from build123d import *

# Parameters (mm, degrees)
F0_R     = 0.635
F0_R_2   = 1.015
F1_DEPTH = 1.85
F2_W     = 2.096224
F2_H     = 1.321533
F3_DEPTH = 0.95


with BuildPart() as f1:
    # F0 (on Top) → F1 (new body)
    with BuildSketch(Plane.XY):
        with BuildLine():
            ThreePointArc((-2.54, -13.97), (-1.796051, -15.766051), (0, -16.51))
            Line((0, -16.51), (12.7, -16.51))
            ThreePointArc((12.7, -16.51), (14.496051, -15.766051), (15.24, -13.97))
            Line((15.24, -13.97), (15.24, 0))
            ThreePointArc((15.24, 0), (14.496051, 1.796051), (12.7, 2.54))
            Line((12.7, 2.54), (0, 2.54))
            ThreePointArc((0, 2.54), (-1.796051, 1.796051), (-2.54, 0))
            Line((-2.54, 0), (-2.54, -13.97))
        make_face()
        with Locations((-1.27, -13.97)):
            Circle(F0_R, mode=Mode.SUBTRACT)
        with Locations((1.27, -13.97)):
            Circle(F0_R, mode=Mode.SUBTRACT)
        with Locations((3.81, -13.97)):
            Circle(F0_R, mode=Mode.SUBTRACT)
        with Locations((6.35, -13.97)):
            Circle(F0_R, mode=Mode.SUBTRACT)
        with Locations((8.89, -13.97)):
            Circle(F0_R, mode=Mode.SUBTRACT)
        with Locations((11.43, -13.97)):
            Circle(F0_R, mode=Mode.SUBTRACT)
        with Locations((13.97, -13.97)):
            Circle(F0_R, mode=Mode.SUBTRACT)
        Circle(F0_R_2, mode=Mode.SUBTRACT)
        with Locations((12.7, 0)):
            Circle(F0_R_2, mode=Mode.SUBTRACT)
    extrude(amount=F1_DEPTH)

    # F2 (on face) → F3 (join)
    with BuildSketch(Plane.XY.offset(1.85)):
        with Locations((5.915654, -5.278095)):
            Rectangle(F2_W, F2_H)
    extrude(amount=F3_DEPTH)


solid = f1.part
Verification items for the finished model (mm, model axes). A direction names the side the tool comes from. Give positions to 0.01 mm unless a question says otherwise; leave off trailing zeros. Write each loop counter-clockwise with the first axis right and the second up, starting at its lowest first coordinate (ties: lowest second). Pieces come first, ordered by that corner, then holes. Notation, with made-up numbers: M -4,-24.5 L 11,-24.5 A25 ccw 11,1.5 Z; hole C 77.25,-13 d11. An arc over 180 degrees is marked long. Put each result on its own line as item: value. Start each with the question number.
1. Section check C-C (y = -0.25). Record the cut outline in (x, z), and give its area (3 significant figures).
2. Section check B-B (z = 0.8). Give the number of separate pieces and of enclosed holes in the cut face, and give its area (3 significant figures).
3. Set-up check for faces 5 (the face through (4.868, -5, 2)), 6 (the face through (5.9, -4.617, 2.3)), 7 (the face through (5.9, -5.939, 2.3)): record each of +Z, -Z, +X, -X, +Y, -Y from which the full face is reachable in a straight line by a thin tool's end or side.
4. Go/stop test with flat-tipped pins: pin 1 Ø2.5 at (x, y) = (12.7, 0) entering from +Z; pin 2 Ø1.2 at (x, y) = (0, 0) entering from -Z; pin 3 Ø1 at (x, z) = (5.5, 2.5) entering from -Y; pin 4 Ø0.5 at (y, z) = (-5.5, 2.5) entering from -X. Record where each tip stops, or that it passes through.
5. Scan lines: line 1 along Y through (x, z) = (3.81, 1.4) (3 decimals); line 2 along Z through (x, y) = (2.75, -12.75); line 3 along Y through (x, z) = (14.5, 0.4). Record each from-to range of solid material in increasing order. Write a range as [from, to].
6. Section check D-D (x = 9.25). Record the cut outline in (y, z).
7. Section check A-A (x = 1.27). Record the cut outline in (y, z) (3 decimals).
8. Draft check along Y on faces 1 (the face through (-2.54, -7, 1)), 2 (the face through (-1.776, 1.816, 0.912)), 3 (the face through (-1.35, -13.34, 0.91)), 4 (the face through (6.691, -13.435, 0.912)). Enter one of: +Y half, -Y half, draft (parallel to the pull), parting line (faces both ways), or undercut.
Answer list:
1. outline: M -2.54,0 L -0.98,0 L -0.98,1.85 L -2.54,1.85 Z; M 0.98,0 L 11.72,0 L 11.72,1.85 L 0.98,1.85 Z; M 13.68,0 L 15.24,0 L 15.24,1.85 L 13.68,1.85 Z
1. area: 25.6 mm2
2. separate pieces: 1
2. enclosed holes: 9
2. area: 318 mm2
3. face 5: +Z, -X, +Y, -Y
3. face 6: +Z, +X, -X, +Y
3. face 7: +Z, +X, -X, -Y
4. pin 1: z = 1.85
4. pin 2: through
4. pin 3: y = -5.94
4. pin 4: x = 4.87
5. line 1: [-16.51, -14.605], [-13.335, 2.54]
5. line 2: [0, 1.85]
5. line 3: [-15.76, -14.32], [-13.62, 1.79]
6. outline: M -16.51,0 L -14.49,0 L -14.49,1.85 L -16.51,1.85 Z; M -13.45,0 L 2.54,0 L 2.54,1.85 L -13.45,1.85 Z
7. outline: M -16.51,0 L -14.605,0 L -14.605,1.85 L -16.51,1.85 Z; M -13.335,0 L 2.54,0 L 2.54,1.85 L -13.335,1.85 Z
8. face 1: draft
8. face 2: +Y half
8. face 3: undercut
8. face 4: undercut
